Verification items for the finished model (mm, model axes). A direction names the side the tool comes from. Round coordinates to 2 decimals unless told otherwise and drop trailing zeros. Write each loop counter-clockwise with the first axis right and the second up, starting at its lowest first coordinate (ties: lowest second). Pieces come first, ordered by that corner, then holes. Notation, with made-up numbers: (37.5, 40) - (87.5, 40) arc R19 cw to (87.5, 56) - close; hole circle Ø7 at (22.5, 51). An arc over 180 degrees is marked (long way). Answer as a JSON object with one key per item and string values.
Autodesk Inventor part; units mm, degrees
ref_plane "YZ Plane" through (0, 0, 0) normal (1, 0, 0) x (0, 1, 0)
ref_plane "XZ Plane" through (0, 0, 0) normal (0, 1, 0) x (-1, 0, 0)
ref_plane "XY Plane" through (0, 0, 0) normal (0, 0, 1) x (1, 0, 0)
sketch "Esquisse2" plane through (0, 0, 0) normal (0, 0, 1) x (1, 0, 0)
  line L0 (-26, -17.5) -> (26, -17.5)
  line L1 (26, -17.5) -> (26, 17.5)
  line L2 (26, 17.5) -> (-26, 17.5)
  line L3 (-26, 17.5) -> (-26, -17.5)
  line L4 (-26, -17.5) -> (26, 17.5) construction
  line L5 (26, -17.5) -> (-26, 17.5) construction
  point P0 (0, 0)
  dimension "d0" = 52
  dimension "d1" = 35
extrude "Extrusion1" add sketch "Esquisse2" along normal blind 5
sketch "Esquisse3" plane through (26, -17.5, 0) normal (1, 0, 0) x (0, 0, -1)
  line L0 (0, 0) -> (0, 35) construction
  line L1 (0, 35) -> (-5, 35) construction
  line L2 (-5, 0) -> (-5, 35) construction
  line L3 (0, 0) -> (-5, 0) construction
  line L4 (0, 17.5) -> (-2.5, 17.5) construction
  line L5 (-1.75, 0) -> (-3.25, 0)
  line L6 (-3.25, 0) -> (-3.25, 35)
  line L7 (-3.25, 35) -> (-1.75, 35)
  line L8 (-1.75, 35) -> (-1.75, 0)
  line L9 (-1.75, 0) -> (-3.25, 35) construction
  line L10 (-3.25, 0) -> (-1.75, 35) construction
  dimension "d4" = 2.5
  dimension "d5" = 1.5
extrude "Extrusion2" add sketch "Esquisse3" along normal blind 1.5
mirror "Symétrie1" about plane through (0, 0, 0) normal (1, 0, 0) of "Extrusion2"
sketch "Esquisse4" plane through (0, 0, 5) normal (0, 0, 1) x (1, 0, 0)
  line L0 (-26, 17.5) -> (-26, -17.5) construction
  line L1 (-26, -17.5) -> (26, -17.5) construction
  line L2 (26, -17.5) -> (26, 17.5) construction
  line L3 (26, 17.5) -> (-26, 17.5) construction
  line L4 (-26, -17.5) -> (26, -17.5)
  line L5 (26, -17.5) -> (26, -10)
  line L6 (26, -10) -> (-26, -10)
  line L7 (-26, -10) -> (-26, -17.5)
  point P0 (0, 0)
  dimension "d8" = 7.5
extrude "Extrusion3" add sketch "Esquisse4" along normal blind 5
sketch "Esquisse5" plane through (-26, 17.5, 0) normal (0, 1, 0) x (1, 0, 0)
  line L0 (52, 0) -> (0, 0) construction
  line L1 (0, 0) -> (0, -1.75) construction
  line L2 (0, -1.75) -> (-1.5, -1.75) construction
  line L3 (-1.5, -1.75) -> (-1.5, -3.25) construction
  line L4 (0, -3.25) -> (-1.5, -3.25) construction
  line L5 (0, -3.25) -> (0, -5) construction
  line L6 (52, -5) -> (0, -5) construction
  line L7 (52, -3.25) -> (52, -5) construction
  line L8 (52, -3.25) -> (53.5, -3.25) construction
  line L9 (53.5, -1.75) -> (53.5, -3.25) construction
  line L10 (52, -1.75) -> (53.5, -1.75) construction
  line L11 (52, 0) -> (52, -1.75) construction
  line L12 (26, 2) -> (26, -12) construction
  line L13 (-12.5, 0) -> (64.5, 0) construction
  line L14 (26, 0) -> (30, 0) construction
  line L15 (30, 0) -> (22, 0)
  line L16 (22, 0) -> (22, -3)
  line L17 (22, -3) -> (30, -3)
  line L18 (30, -3) -> (30, 0)
  dimension "d11" = 4
  dimension "d12" = 8
  dimension "d13" = 3
extrude "Extrusion4" add sketch "Esquisse5" along normal blind 8
fillet "Congé1" radius 2 2 edges at (4, 25.5, 1.5) (-4, 25.5, 1.5)
fillet "Congé1" radius 4 2 edges at (0, -17.5, 0) (0, -10, 5)
sketch "Esquisse6" plane through (-4, 17.5, 3) normal (0, 0, 1) x (1, 0, 0)
  line L0 (30, -23.5) -> (-22, -23.5) construction
  line L1 (30, -23.5) -> (30, 0) construction
  line L2 (30, 0) -> (-22, 0) construction
  line L3 (-22, 0) -> (-22, -23.5) construction
  arc A0 (2, 8) -> (0, 6) centre (2, 6) ccw construction
  line L4 (0, 0) -> (0, 6) construction
  line L5 (8, 0) -> (0, 0) construction
  line L6 (8, 0) -> (8, 6) construction
  arc A1 (8, 6) -> (6, 8) centre (6, 6) ccw construction
  line L7 (2, 8) -> (6, 8) construction
  line L8 (4, 0) -> (4, 4) construction
  circle A2 centre (4, 4) radius 2
  point P0 (4, -17.5)
  dimension "d18" = 4
  dimension "d19" = 4
extrude "Extrusion5" cut sketch "Esquisse6" against normal through all
properties part number "A3_BatteriesTray" material "Plastique ABS"
1. Material ranges on probe 1 along Z at (x, y) = (-10, -0.5); probe 2 along Y at (x, z) = (-0.5, 4.5); probe 3 along Y at (x, z) = (-1.5, 1.5), recorded low to high. Write a range as from..to.
Completed:
{"probe 1": "z = 0..5", "probe 2": "y = -17.5..17.5", "probe 3": "y = -16.62..20.18, 22.82..25.5"}
2. Cross-section at A-A (x = 0). Record the boundary of the cut face in (y, z).
Completed:
{"outline": "(-17.5, 4) arc R4 ccw to (-13.5, 0) - (19.5, 0) - (19.5, 3) - (17.5, 3) - (17.5, 5) - (-6, 5) arc R4 cw to (-10, 9) - (-10, 10) - (-17.5, 10) - close; (23.5, 0) - (25.5, 0) - (25.5, 3) - (23.5, 3) - close"}
3. Go/stop test with flat-tipped pins: pin 1 (8 mm diameter, centred on x = 6.5, y = 12.5, fed in from +Z); pin 2 (4 mm diameter, centred on y = 9.5, z = 8.5, fed in from -X); pin 3 (0.9 mm diameter, centred on y = 21.5, z = 1.5, fed in from -X); pin 4 (4.5 mm diameter, centred on x = 0, y = 21.5, fed in from +Z). Record where each tip stops, or that it passes through.
Completed:
{"pin 1": "stops at z = 5", "pin 2": "passes through", "pin 3": "stops at x = -4", "pin 4": "stops at z = 3"}
4. Access from +Z, -Z, +X, -X, +Y, -Y to the whole of each face (thin tool, end or side, straight path). Record for faces 1 (the face through (27, 0, 3.25)), 2 (the face through (-26, -8, 5)), 3 (the face through (-4, 20, 1)), 4 (the face through (-26, 1, 1)).
Completed:
{"face 1": "+Z, +X, +Y, -Y", "face 2": "+Z, -X, +Y, -Y", "face 3": "+Z, -Z, -X, +Y", "face 4": "-Z, -X, +Y, -Y"}
5. Mould release check, pull along Y, two halves, no side actions. Record for faces 5 (the face through (3.4, 24.93, 1.48)), 6 (the face through (0, 6, 5)), 7 (the face through (-0.26, 23.483, 1.521)), 8 (the face through (0, -17.5, 7)): released by +Y, released by -Y, zero draft, split by the parting line, or undercut.
Completed:
{"face 5": "released by +Y", "face 6": "zero draft", "face 7": "undercut", "face 8": "released by -Y"}
6. Cross-section at B-B (y = 21.5). Record the boundary of the cut face in (x, z), plus the area to 3 significant figures.
Completed:
{"outline": "(-4, 0) - (-2, 0) - (-2, 3) - (-4, 3) - close; (2, 0) - (4, 0) - (4, 3) - (2, 3) - close", "area": "12.0 mm^2"}
7. Cross-section at D-D (y = 11.5). Record the boundary of the cut face in (x, z), plus the area to 4 significant figures.
Completed:
{"outline": "(-27.5, 1.75) - (-26, 1.75) - (-26, 0) - (26, 0) - (26, 1.75) - (27.5, 1.75) - (27.5, 3.25) - (26, 3.25) - (26, 5) - (-26, 5) - (-26, 3.25) - (-27.5, 3.25) - close", "area": "264.5 mm^2"}
8. Cross-section at C-C (x = -23). Record the boundary of the cut face in (y, z), plus the area to 4 significant figures.
Completed:
{"outline": "(-17.5, 4) arc R4 ccw to (-13.5, 0) - (17.5, 0) - (17.5, 5) - (-6, 5) arc R4 cw to (-10, 9) - (-10, 10) - (-17.5, 10) - close", "area": "212.5 mm^2"}
